```python
from build123d import *

# Parameters (mm, degrees)
SKETCH1_R           = 32.8295
SKETCH1_R_2         = 2.921000021
SKETCH1_W           = 6.35
SKETCH1_H           = 40.5892
BOSS_EXTRUDE1_DEPTH = 3.4036


with BuildPart() as part:
    # Sketch1 → Boss-Extrude1 (new body)
    with BuildSketch(Plane.XY):
        with BuildLine():
            Line((6310.72013516, 3386.676584946), (6310.72013516, 3341.108984946))
            Line((6310.72013516, 3341.108984946), (6304.37013516, 3341.108984946))
            Line((6304.37013516, 3341.108984946), (6304.37013516, 3328.408984946))
            Line((6304.37013516, 3328.408984946), (6310.72013516, 3328.408984946))
            Line((6310.72013516, 3328.408984946), (6356.849906468, 3325.851217453))
            ThreePointArc((6356.849906468, 3325.851217453), (6360.439847706, 3325.821566173), (6364.016642615, 3326.129941694))
            Line((6364.016642615, 3326.129941694), (6399.62013516, 3330.898184946))
            Line((6399.62013516, 3330.898184946), (6710.77013516, 3330.898184946))
            Line((6710.77013516, 3330.898184946), (6710.77013516, 3343.598184946))
            Line((6710.77013516, 3343.598184946), (6704.42013516, 3343.598184946))
            Line((6704.42013516, 3343.598184946), (6704.42013516, 3384.187384946))
            Line((6704.42013516, 3384.187384946), (6710.77013516, 3384.187384946))
            Line((6710.77013516, 3384.187384946), (6710.77013516, 3396.887384946))
            Line((6710.77013516, 3396.887384946), (6399.62013516, 3396.887384946))
            Line((6399.62013516, 3396.887384946), (6364.016642615, 3401.655628197))
            ThreePointArc((6364.016642615, 3401.655628197), (6360.439847706, 3401.964003719), (6356.849906468, 3401.934352439))
            Line((6356.849906468, 3401.934352439), (6310.72013516, 3399.376584946))
            Line((6310.72013516, 3399.376584946), (6304.37013516, 3399.376584946))
            Line((6304.37013516, 3399.376584946), (6304.37013516, 3386.676584946))
            Line((6304.37013516, 3386.676584946), (6310.72013516, 3386.676584946))
        make_face()
        with Locations((6358.95920556, 3363.892784946)):
            Circle(SKETCH1_R, mode=Mode.SUBTRACT)
        with Locations((6327.70875532, 3342.097845648)):
            Circle(SKETCH1_R_2, mode=Mode.SUBTRACT)
        with Locations((6390.168898653, 3342.039522577)):
            Circle(SKETCH1_R_2, mode=Mode.SUBTRACT)
        with Locations((6390.127285576, 3385.805356845)):
            Circle(SKETCH1_R_2, mode=Mode.SUBTRACT)
        with Locations((6327.749512467, 3385.746047315)):
            Circle(SKETCH1_R_2, mode=Mode.SUBTRACT)
        with Locations((6402.79513516, 3363.892784946)):
            Rectangle(SKETCH1_W, SKETCH1_H, mode=Mode.SUBTRACT)
        with BuildLine():
            Line((6421.84513516, 3353.123184946), (6421.84513516, 3374.662384946))
            ThreePointArc((6421.84513516, 3374.662384946), (6423.705007099, 3379.152513006), (6428.19513516, 3381.012384946))
            Line((6428.19513516, 3381.012384946), (6523.44513516, 3381.012384946))
            ThreePointArc((6523.44513516, 3381.012384946), (6527.93526322, 3379.152513006), (6529.79513516, 3374.662384946))
            Line((6529.79513516, 3374.662384946), (6529.79513516, 3353.123184946))
            ThreePointArc((6529.79513516, 3353.123184946), (6527.93526322, 3348.633056885), (6523.44513516, 3346.773184946))
            Line((6523.44513516, 3346.773184946), (6428.19513516, 3346.773184946))
            ThreePointArc((6428.19513516, 3346.773184946), (6423.705007099, 3348.633056885), (6421.84513516, 3353.123184946))
        make_face(mode=Mode.SUBTRACT)
        with BuildLine():
            Line((6682.19513516, 3381.012384946), (6574.24513516, 3381.012384946))
            ThreePointArc((6574.24513516, 3381.012384946), (6569.755007099, 3379.152513006), (6567.89513516, 3374.662384946))
            Line((6567.89513516, 3374.662384946), (6567.89513516, 3353.123184946))
            ThreePointArc((6567.89513516, 3353.123184946), (6569.755007099, 3348.633056885), (6574.24513516, 3346.773184946))
            Line((6574.24513516, 3346.773184946), (6682.19513516, 3346.773184946))
            ThreePointArc((6682.19513516, 3346.773184946), (6686.68526322, 3348.633056885), (6688.54513516, 3353.123184946))
            Line((6688.54513516, 3353.123184946), (6688.54513516, 3374.662384946))
            ThreePointArc((6688.54513516, 3374.662384946), (6686.68526322, 3379.152513006), (6682.19513516, 3381.012384946))
        make_face(mode=Mode.SUBTRACT)
        with Locations((6548.84513516, 3363.892784946)):
            Rectangle(SKETCH1_W, SKETCH1_H, mode=Mode.SUBTRACT)
    extrude(amount=BOSS_EXTRUDE1_DEPTH)


solid = part.part
```
Here's how the part is built. I have some questions about the finished solid (model axes, mm). A direction names the side the tool comes from. Coordinates: 2 decimals unless noted, no trailing zeros. Loops run counter-clockwise (first coordinate to the right, second up) from the corner with the lowest first, then second, coordinate; pieces in that order, holes last. Notation, with made-up numbers: (82.5, 35.5) - (134.5, 35.5) arc R12 ccw to (134.5, 44.5) - close; hole circle Ø2 at (45.5, 20.5). An arc over 180 degrees is marked (long way). Return JSON: item names as keys, results as strings. Group by question number.
Item 1: Will these pins go through, and if not, where does the flat tip stop? P1, Ø1, axis at x = 6499, z = 1.5, coming from the -Y side; P2, Ø1.5, axis at y = 3372.5, z = 0.5, coming from the -X side; P3, Ø1, axis at x = 6497, z = 1.5, coming from the +Y side.
Item 2: If we section it at A-A on x = 6674: Write out the boundary of the cut face in (y, z).
Item 3: If we section it at C-C on x = 6334.5: Write out the boundary of the cut face in (y, z), and give its area (3 significant figures).
Item 4: I need wall thicknesses on line 1 (Y direction, x = 6668, z = 2.6); line 2 (X direction, y = 3388, z = 2.9); line 3 (X direction, y = 3367, z = 3.05). Which ranges of each line are inside material? Lowest first, please. Write a range as from..to.
Item 5: We'd pull the mould along X, two halves only. Please class faces 1 (the face through (6459.6, 3381.4, 3.404)), 2 (the face through (6569.805, 3379.202, 1.678)): +X half, -X half, draft (parallel to the pull), parting line (faces both ways), or undercut.
Item 6: On a 3-axis mill with a long thin cutter (end or side, diameter ignored), from which of +Z, -Z, +X, -X, +Y, -Y can I reach the whole of each face in a straight line? I mean faces 3 (the face through (6423.755, 3348.584, 1.678)), 4 (the face through (6459.6, 3381.4, 0)). Say none if no direction works.
Item 7: If we section it at D-D on x = 6560: Write out the boundary of the cut face in (y, z).
Item 8: If we section it at B-B on y = 3369: Write out the boundary of the cut face in (x, z).
Calculated:
{
 "1": {"P1": "stops at y = 3330.9", "P2": "stops at x = 6310.72", "P3": "stops at y = 3396.89"},
 "2": {"outline": "(3330.9, 0) - (3346.77, 0) - (3346.77, 3.4) - (3330.9, 3.4) - close; (3381.01, 0) - (3396.89, 0) - (3396.89, 3.4) - (3381.01, 3.4) - close"},
 "3": {"outline": "(3327.09, 0) - (3341.99, 0) - (3341.99, 3.4) - (3327.09, 3.4) - close; (3385.79, 0) - (3400.7, 0) - (3400.7, 3.4) - (3385.79, 3.4) - close", "area": "101 mm^2"},
 "4": {"line 1": "y = 3330.9..3346.77, 3381.01..3396.89", "line 2": "x = 6304.37..6325.89, 6329.61..6336.67, 6381.24..6388.2, 6392.05..6710.77", "line 3": "x = 6310.72..6326.28, 6391.64..6399.62, 6405.97..6421.85, 6529.8..6545.67, 6552.02..6567.9, 6688.55..6704.42"},
 "5": {"face 1": "draft", "face 2": "undercut"},
 "6": {"face 3": "+Z, -Z", "face 4": "-Z, +X, -X, +Y, -Y"},
 "7": {"outline": "(3330.9, 0) - (3396.89, 0) - (3396.89, 3.4) - (3330.9, 3.4) - close"},
 "8": {"outline": "(6310.72, 0) - (6326.53, 0) - (6326.53, 3.4) - (6310.72, 3.4) - close; (6391.39, 0) - (6399.62, 0) - (6399.62, 3.4) - (6391.39, 3.4) - close; (6405.97, 0) - (6421.85, 0) - (6421.85, 3.4) - (6405.97, 3.4) - close; (6529.8, 0) - (6545.67, 0) - (6545.67, 3.4) - (6529.8, 3.4) - close; (6552.02, 0) - (6567.9, 0) - (6567.9, 3.4) - (6552.02, 3.4) - close; (6688.55, 0) - (6704.42, 0) - (6704.42, 3.4) - (6688.55, 3.4) - close"}
}
